```python
from build123d import *

# Parameters (mm, degrees)
SKETCH1_R      = 1
EXTRUDE1_DEPTH = 2


with BuildPart() as part:
    # Sketch1 → Extrude1 (new body)
    with BuildSketch(Plane.XY):
        with BuildLine():
            Line((-12.5, 33.957513111), (-12.5, 26.457513111))
            Line((-12.5, 26.457513111), (-18.696787712, 20.166311741))
            Line((-18.696787712, 20.166311741), (-20.446699126, 18.389738847))
            ThreePointArc((-20.446699126, 18.389738847), (0, -27.5), (20.446699126, 18.389738847))
            Line((20.446699126, 18.389738847), (18.696787712, 20.166311741))
            Line((18.696787712, 20.166311741), (12.5, 26.457513111))
            Line((12.5, 26.457513111), (12.5, 33.957513111))
            Line((12.5, 33.957513111), (7.5, 33.957513111))
            Line((7.5, 33.957513111), (7.5, 21.213203436))
            ThreePointArc((7.5, 21.213203436), (0, -22.5), (-7.5, 21.213203436))
            Line((-7.5, 21.213203436), (-7.5, 33.957513111))
            Line((-7.5, 33.957513111), (-12.5, 33.957513111))
        make_face()
        with Locations(Location((-10, 30, 0), (0, 0, 180))):
            Circle(SKETCH1_R, mode=Mode.SUBTRACT)
        with Locations(Location((10, 30, 0), (0, 0, 180))):
            Circle(SKETCH1_R, mode=Mode.SUBTRACT)
    extrude(amount=EXTRUDE1_DEPTH)


solid = part.part
```
Verification items for the finished model (mm, model axes). A direction names the side the tool comes from. Give positions to 0.01 mm unless a question says otherwise; leave off trailing zeros. Order: outer loops, then holes, each group sorted by start corner. A loop starts at its lowest first (then second) coordinate and runs counter-clockwise, first axis right, second up. Notation, with made-up numbers: (83, 75) -> (131, 75) arc R13 ccw to (131, 81) -> close; hole circle Ø2 at (2, 24.5). An arc over 180 degrees is marked (long way). One line per item, written item: value.
(1) Sectioned sample at A-A on y = 0. Record the cut outline in (x, z), then the cut area to 3 significant figures.
Final values:
outline: (-27.5, 0) -> (-22.5, 0) -> (-22.5, 2) -> (-27.5, 2) -> close; (22.5, 0) -> (27.5, 0) -> (27.5, 2) -> (22.5, 2) -> close
area: 20.0 mm^2
(2) Scan lines: line 1 along X through (y, z) = (30, 1.6); line 2 along X through (y, z) = (0, 0.5); line 3 along Y through (x, z) = (10, 0.65). Record each from-to range of solid material in increasing order. Write a range as [from, to].
Final values:
line 1: [-12.5, -11], [-9, -7.5], [7.5, 9], [11, 12.5]
line 2: [-27.5, -22.5], [22.5, 27.5]
line 3: [-25.62, -20.16], [20.16, 29], [31, 33.96]
(3) Draft check along X on faces 1 (the face through (12.5, 30, 1)), 2 (the face through (10, 33.958, 1)), 3 (the face through (7.5, 28, 1)). Enter one of: pulls with the +X half, pulls with the -X half, needs draft (parallel to the pull), parting line crosses it, or undercut.
Final values:
face 1: pulls with the +X half
face 2: needs draft
face 3: undercut
(4) Gauge pin test, flat ends, axial feed: pin 1 (1 mm diameter, centred on y = 30.5, z = 1, fed in from +X); pin 2 (1 mm diameter, centred on y = -15, z = 0.5, fed in from -X); pin 3 (12 mm diameter, centred on x = -11.5, y = 6, fed in from +Z); pin 4 (1 mm diameter, centred on y = 22.5, z = 0.5, fed in from -X). Record the tip position at first contact, or that the pin passes through.
Final values:
pin 1: x = 12.5
pin 2: x = -23.37
pin 3: through
pin 4: x = -16.89
(5) Sectioned sample at C-C on z = 0.45. Record the cut outline in (x, y), then the cut area to 3 significant figures.
Final values:
outline: (-20.45, 18.39) arc R27.5 ccw (long way) to (20.45, 18.39) -> (12.5, 26.46) -> (12.5, 33.96) -> (7.5, 33.96) -> (7.5, 21.21) arc R22.5 cw (long way) to (-7.5, 21.21) -> (-7.5, 33.96) -> (-12.5, 33.96) -> (-12.5, 26.46) -> close; hole circle Ø2 at (-10, 30); hole circle Ø2 at (10, 30)
area: 796 mm^2
(6) Tool access check on faces 4 (the face through (-8, 22, 0)), 5 (the face through (-7.5, 27, 1)), 6 (the face through (-12.5, 30, 1)). Record the directions out of +Z, -Z, +X, -X, +Y, -Y that give a thin tool (end or side, any length) a straight path to the whole face; none if there is none.
Final values:
face 4: -Z, +X, -X, +Y, -Y
face 5: +Z, -Z, +Y
face 6: +Z, -Z, -X, +Y
(7) Sectioned sample at B-B on x = 17. Record the cut outline in (y, z).
Final values:
outline: (-21.62, 0) -> (-14.74, 0) -> (-14.74, 2) -> (-21.62, 2) -> close; (14.74, 0) -> (21.89, 0) -> (21.89, 2) -> (14.74, 2) -> close
(8) Sectioned sample at D-D on x = 10. Record the cut outline in (y, z), then the cut area to 3 significant figures.
Final values:
outline: (-25.62, 0) -> (-20.16, 0) -> (-20.16, 2) -> (-25.62, 2) -> close; (20.16, 0) -> (29, 0) -> (29, 2) -> (20.16, 2) -> close; (31, 0) -> (33.96, 0) -> (33.96, 2) -> (31, 2) -> close
area: 34.5 mm^2
